from build123d import *
from build123d.topology import SkipClean

# Parameters (mm, degrees)
CROQUIS1_R                          = 13
CROQUIS1_R_2                        = 11.05
SALIENTE_EXTRUIR1_DEPTH             = 1
BARRER_L_MINA1_PROFILE_R            = 13.05
BARRER_L_MINA1_PROFILE_R_2          = 11.05
CROQUIS35_R                         = 13
CROQUIS35_R_2                       = 11.05
SALIENTE_EXTRUIR3_DEPTH             = 15
SALIENTE_EXTRUIR3_DIRECTION_2_REACH = 73.094
CORTAR_EXTRUIR1_REACH               = 80.217
CROQUIS37_R                         = 11.05


with BuildPart() as part:
    # Croquis1 → Saliente-Extruir1 (new body)
    with BuildSketch(Plane(origin=(0, 0, 0), x_dir=(1, 0, 0), z_dir=(0, 1, 0))):
        with Locations(Location((0, 0, 0), (0, 0, 270))):
            Circle(CROQUIS1_R)
        with Locations(Location((0, 0, 0), (0, 0, 270))):
            Circle(CROQUIS1_R_2, mode=Mode.SUBTRACT)
    extrude(amount=SALIENTE_EXTRUIR1_DEPTH)

    # Barrer-L_mina1: sweep along a path in Croquis2
    with BuildLine(Plane.XY) as barrer_l_mina1_path:
        Line((0, 1), (0, 22))
        ThreePointArc((0, 22), (2.241962153, 29.88875594), (8.297662704, 35.41933958))
        Line((8.297662704, 35.41933958), (27.084738117, 44.802611794))
    # Barrer-L_mina1 profile (on start of the path) → Barrer-L_mina1 (sweep)
    with BuildSketch(Plane.ZX.offset(1)):
        Circle(BARRER_L_MINA1_PROFILE_R)
        Circle(BARRER_L_MINA1_PROFILE_R_2, mode=Mode.SUBTRACT)
    sweep(path=barrer_l_mina1_path.line)

    # Croquis35 → Saliente-Extruir3 (add)
    with BuildSketch(Plane(origin=(0, 0, -14.9), x_dir=(-1, 0, 0), z_dir=(0, 0, -1))):
        with Locations((0, 13)):
            Circle(CROQUIS35_R)
        with Locations((0, 13)):
            Circle(CROQUIS35_R_2, mode=Mode.SUBTRACT)
    saliente_extruir3 = extrude(amount=SALIENTE_EXTRUIR3_DEPTH)

    # Croquis35 → Saliente-Extruir3 direction 2 (add, up to next)
    with BuildSketch(Plane(origin=(0, 0, -14.9), x_dir=(-1, 0, 0), z_dir=(0, 0, -1)), mode=Mode.PRIVATE) as saliente_extruir3_direction_2_sk1:
        with Locations((0, 13)):
            Circle(CROQUIS35_R)
        with Locations((0, 13)):
            Circle(CROQUIS35_R_2, mode=Mode.SUBTRACT)
    saliente_extruir3_direction_2_tool1 = extrude(saliente_extruir3_direction_2_sk1.sketch, amount=-SALIENTE_EXTRUIR3_DIRECTION_2_REACH, mode=Mode.PRIVATE) - part.part
    saliente_extruir3_direction_2 = saliente_extruir3_direction_2_tool1.solids().sort_by_distance((12.632304, 13, -14.9))[0]
    add(saliente_extruir3_direction_2)

    # Croquis37 → Cortar-Extruir1 (cut, up to next)
    with BuildSketch(Plane(origin=(0, 0, -29.9), x_dir=(-1, 0, 0), z_dir=(0, 0, -1)), mode=Mode.PRIVATE) as cortar_extruir1_sk1:
        with Locations((0, 13)):
            Circle(CROQUIS37_R)
    cortar_extruir1_tool1 = extrude(cortar_extruir1_sk1.sketch, amount=-CORTAR_EXTRUIR1_REACH, mode=Mode.PRIVATE) & part.part
    cortar_extruir1 = cortar_extruir1_tool1.solids().sort_by_distance((0, 13, -29.9))[0]
    add(cortar_extruir1, mode=Mode.SUBTRACT)

    # Simetr_a1: Saliente-Extruir3, Saliente-Extruir3 direction 2, Cortar-Extruir1 across plane
    with SkipClean():  # the faces are left unmerged after this step: merging them gives an invalid solid
        add(saliente_extruir3.mirror(Plane.XY))
        add(saliente_extruir3_direction_2.mirror(Plane.XY))
        add(cortar_extruir1.mirror(Plane.XY), mode=Mode.SUBTRACT)


solid = part.part
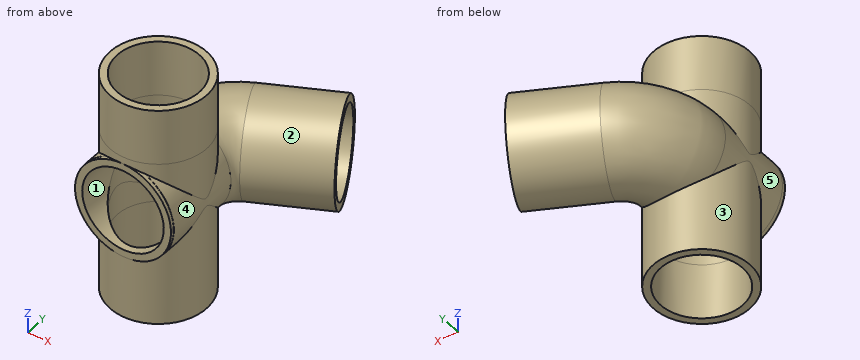
Design review of the part built by this model. Coordinates are the model's own, in mm. Face numbers are marked on the shaded views. A direction names the side the tool comes from. Give positions to 0.01 mm unless a question says otherwise; leave off trailing zeros. Write each loop counter-clockwise with the first axis right and the second up, starting at its lowest first coordinate (ties: lowest second). Pieces come first, ordered by that corner, then holes. Notation, with made-up numbers: M -28,34.25 L -14,34.25 A30 ccw -14,73.25 Z; hole C 77,-16 d4. An arc over 180 degrees is marked long. Return JSON: item names as keys, results as strings. Group by question number.
Item 1: Wall thickness on line 1 along Y through (x, z) = (0, -25.25); line 2 along X through (y, z) = (13, -10.5); line 3 along Y through (x, z) = (-6.5, -20.5): over which ranges is each line inside the solid? List them lowest first.
Item 2: Take a section at B-B (y = 11.5). Give the boundary of the cut face in (x, z), plus the area to 3 significant figures.
Item 3: Take a section at A-A (z = -3). Give the boundary of the cut face in (x, y), plus the area to 3 significant figures.
Item 4: Take a section at C-C (z = 22). Give the boundary of the cut face in (x, y).
Item 5: The part is to be moulded in two halves that separate along Z. For the marked faces 1, 2 and 3, say which applies: pulls with the +Z half, pulls with the -Z half, needs draft (parallel to the pull), parting line crosses it, or undercut.
Item 6: Tool access review of the marked faces 4 and 5: name each direction out of +Z, -Z, +X, -X, +Y, -Y from which nothing blocks a thin tool from reaching the whole face with its end or side.
Item 7: Clearance check with flat-ended pins moving along their axes: pin 1 Ø8 at (x, y) = (26, 49) entering from +Z; pin 2 Ø8 at (y, z) = (30.5, 15) entering from -X; pin 3 Ø4 at (y, z) = (10, 15) entering from -X. State where each tip first meets the part, or that it passes through.
Return value:
{
 "1": {"line 1": "y = 0 to 1.95, 24.05 to 26", "line 2": "x = -13 to -11.05, 11.05 to 13", "line 3": "y = 1.74 to 4.06, 21.94 to 24.26"},
 "2": {"outline": "M -12.91,-29.9 L -10.95,-29.9 L -10.95,-1.5 A11.05 cw -10.95,1.5 L -10.95,29.9 L -12.91,29.9 L -12.91,1.88 A13.05 ccw -12.91,-1.88 Z; M 10.95,-29.9 L 12.91,-29.9 L 12.91,-1.88 A13.05 ccw 12.91,1.88 L 12.91,29.9 L 10.95,29.9 L 10.95,1.5 A11.05 cw 10.95,-1.5 Z", "area": "235 mm2"},
 "3": {"outline": "M -12.7,1 L -12.65,1 L -12.65,0 L -10.63,0 L -10.63,10 A11.05 cw -10.63,16 L -10.63,22 A25.63 cw 3.55,44.93 L 22.33,54.32 L 21.41,56.16 L 2.62,46.78 A27.7 ccw -12.7,22 L -12.7,15.77 A13 ccw -12.7,10.23 Z; M 10.63,0 L 12.65,0 L 12.65,1 L 12.7,1 L 12.7,10.23 A13 ccw 12.7,15.77 L 12.7,22 A2.3 cw 13.97,24.06 L 32.76,33.44 L 31.84,35.29 L 13.05,25.91 A4.37 ccw 10.63,22 L 10.63,16 A11.05 cw 10.63,10 Z", "area": "245 mm2"},
 "4": {"outline": "C 0,13 d26; hole C 0,13 d22.1"},
 "5": {"face 1": "undercut", "face 2": "parting line crosses it", "face 3": "needs draft"},
 "6": {"face 4": "+X", "face 5": "-X"},
 "7": {"pin 1": "stops at z = 13.05", "pin 2": "stops at x = -5.5", "pin 3": "stops at x = -12.96"}
}
